from build123d import *

# Parameters (mm, degrees)
F0_W     = 12
F0_H     = 220
F1_DEPTH = 3
F2_R     = 5
F3_R     = 5
F4_R     = 5
F5_R     = 5
F6_R     = 4
F7_DEPTH = 25


with BuildPart() as f1:
    # F0 (on Front) → F1 (new body)
    with BuildSketch(Plane.XZ):
        with Locations((6, 110)):
            Rectangle(F0_W, F0_H)
    extrude(amount=F1_DEPTH)

    # F2
    f2_edges = [f1.edges().sort_by_distance(p)[0] for p in [
        (0, -1.5, 220),
    ]]
    fillet(f2_edges, radius=F2_R)

    # F3
    f3_edges = [f1.edges().sort_by_distance(p)[0] for p in [
        (12, -1.5, 220),
    ]]
    fillet(f3_edges, radius=F3_R)

    # F4
    f4_edges = [f1.edges().sort_by_distance(p)[0] for p in [
        (0, -1.5, 0),
    ]]
    fillet(f4_edges, radius=F4_R)

    # F5
    f5_edges = [f1.edges().sort_by_distance(p)[0] for p in [
        (12, -1.5, 0),
    ]]
    fillet(f5_edges, radius=F5_R)

    # F6 (on face) → F7 (cut)
    with BuildSketch(Plane.XZ.offset(3)):
        with Locations((6, 215)):
            Circle(F6_R)
        with Locations((6, 5)):
            Circle(F6_R)
    extrude(amount=-F7_DEPTH, mode=Mode.SUBTRACT)


solid = f1.part
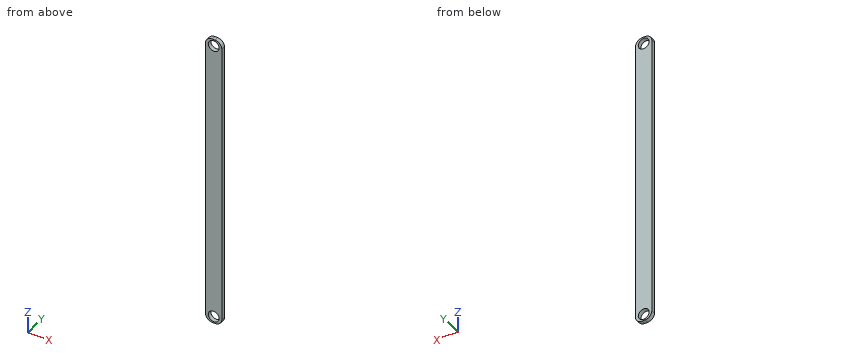
Could you check a few things on this model? Use its own coordinates, in mm. Round coordinates to 2 decimals unless told otherwise and drop trailing zeros. Order: outer loops, then holes, each group sorted by start corner. A loop starts at its lowest first (then second) coordinate and runs counter-clockwise, first axis right, second up.
(1) Please list where these lines run through material, in increasing order: line 1 along Z through (x, y) = (6, -1.3); line 2 along Z through (x, y) = (4, -2.75); line 3 along Z through (x, y) = (0.75, -0.2).
Response values:
line 1: z = 0 to 1, 9 to 211, 219 to 220
line 2: z = 0.1 to 1.54, 8.46 to 211.54, 218.46 to 219.9
line 3: z = 2.37 to 217.63
(2) Imagine slicing it at A-A (y = -2.3). Write out the boundary of the cut face in (x, z).
Response values:
outline: (0, 5) arc R5 ccw to (5, 0) - (7, 0) arc R5 ccw to (12, 5) - (12, 215) arc R5 ccw to (7, 220) - (5, 220) arc R5 ccw to (0, 215) - close; hole circle Ø8 at (6, 5); hole circle Ø8 at (6, 215)
(3) I'm going to push flat-ended pins straight in: pin 1 (1 mm diameter, centred on x = 10, y = -0.5, fed in from +Z); pin 2 (1 mm diameter, centred on x = 9.5, y = -2.5, fed in from -Z). Where does each tip first touch, or does it pass through?
Response values:
pin 1: stops at z = 219.33
pin 2: stops at z = 0.42
